Build history of the part. All positions in model axes, mm. A direction names the side the tool comes from. Round coordinates to 2 decimals unless told otherwise and drop trailing zeros. Use a Markdown table: item, result.
from build123d import *

# Parameters (mm, degrees)
F0_W     = 76.2
F0_H     = 9.525
F1_DEPTH = 9.525
F2_DEPTH = 9.525
F2_TAPER = 12


with BuildPart() as f1:
    # F0 (on Top) → F1 (new body)
    with BuildSketch(Plane.XY):
        with Locations((38.1, -4.7625)):
            Rectangle(F0_W, F0_H)
    extrude(amount=-F1_DEPTH)

    # F0 (on Top) → F2 (join)
    with BuildSketch(Plane.XY):
        with Locations((38.1, -4.7625)):
            Rectangle(F0_W, F0_H)
        Polygon((0, -9.525), (0, 0), (-4.7625, -4.7625), align=None)
    extrude(amount=-F2_DEPTH, taper=F2_TAPER)


solid = f1.part
Q1. Pull direction Z, two halves, no side cores. Call faces 1 (the face through (35, -5, 0)), 2 (the face through (76.2, -5, -5)), 3 (the face through (37, -5, -9.525)): pulls with the +Z half, pulls with the -Z half, needs draft (parallel to the pull), parting line crosses it, or undercut.
Results found:
| item | result |
|---|---|
| face 1 | pulls with the +Z half |
| face 2 | needs draft |
| face 3 | pulls with the -Z half |
Q2. Which spindle directions (+Z, -Z, +X, -X, +Y, -Y) get a long thin tool onto all of the face, cutting with end or side? Do faces 4 (the face through (38, -9.525, -5)), 5 (the face through (0, -1, -7)), 6 (the face through (0, -9, -7)). Say none if no direction does.
Results found:
| item | result |
|---|---|
| face 4 | +Z, -Z, +X, -X, -Y |
| face 5 | -Z, -X, +Y |
| face 6 | -Z, -X, -Y |
Q3. Probe line 1 (X direction, y = -8, z = -5.75); line 2 (X direction, y = -3.75, z = -3). List the from-to ranges inside material, lowest first.
Results found:
| item | result |
|---|---|
| line 1 | x = 0 to 76.2 |
| line 2 | x = -2.85 to 76.2 |
Q4. Drop flat-ended pins along their axis: pin 1 (2.5 mm diameter, centred on y = -2, z = -4, fed in from -X); pin 2 (2.5 mm diameter, centred on y = -8, z = -4, fed in from -X). Give the stop position or say it passes through.
Results found:
| item | result |
|---|---|
| pin 1 | stops at x = -2.1 |
| pin 2 | stops at x = -1.63 |
